Geometry: final body of the model. Coordinates: model frame, mm. Face numbers are marked on the shaded views. A direction names the side the tool comes from. Round coordinates to 2 decimals unless told otherwise and drop trailing zeros. Loops run counter-clockwise (first coordinate to the right, second up) from the corner with the lowest first, then second, coordinate; pieces in that order, holes last. Notation, with made-up numbers: (67, -22.75) -> (90, -22.75) arc R26 ccw to (90, 13.25) -> close; hole circle Ø11 at (-25.75, 60). An arc over 180 degrees is marked (long way). Answer in a Markdown table with one row per item.
```python
from build123d import *

# Parameters (mm, degrees)
SKETCH1_R           = 2.5
BOSS_EXTRUDE1_DEPTH = 15
SKETCH2_R           = 5
BOSS_EXTRUDE2_DEPTH = 3
CUT_EXTRUDE1_START  = -1.5
CUT_EXTRUDE1_DEPTH  = 1.5


with BuildPart() as part:
    # Sketch1 → Boss-Extrude1 (new body)
    with BuildSketch(Plane(origin=(0, 0, 0), x_dir=(1, 0, 0), z_dir=(0, 1, 0))):
        with Locations(Location((0, 0, 0), (0, 0, 270))):
            Circle(SKETCH1_R)
    extrude(amount=BOSS_EXTRUDE1_DEPTH)

    # Sketch2 → Boss-Extrude2 (add)
    with BuildSketch(Plane(origin=(0, 15, 0), x_dir=(1, 0, 0), z_dir=(0, 1, 0))):
        with Locations(Location((0, 0, 0), (0, 0, 270))):
            Circle(SKETCH2_R)
    extrude(amount=BOSS_EXTRUDE2_DEPTH)

    # Sketch3 → Cut-Extrude1 (cut)
    with BuildSketch(Plane(origin=(0, 18, 0), x_dir=(1, 0, 0), z_dir=(0, 1, 0)).offset(CUT_EXTRUDE1_START)):
        with BuildLine():
            Line((-1.5, 4.769696007), (-1.5, -4.769696007))
            ThreePointArc((-1.5, -4.769696007), (0, -5), (1.5, -4.769696007))
            Line((1.5, -4.769696007), (1.5, 4.769696007))
            ThreePointArc((1.5, 4.769696007), (0, 5), (-1.5, 4.769696007))
        make_face()
    extrude(amount=CUT_EXTRUDE1_DEPTH, mode=Mode.SUBTRACT)


solid = part.part
```
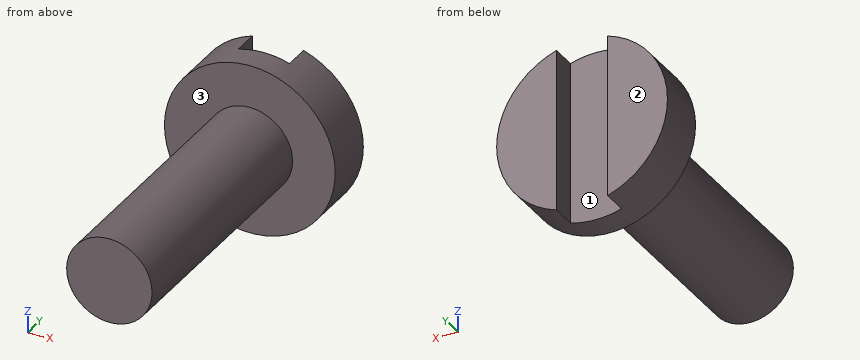
Item 1: Cut plane D-D (y = 9.5). Output: boundary loops of the cut face in (x, z).
Answer:
| item | result |
|---|---|
| outline | circle Ø5 at (0, 0) |
Item 2: Cut plane B-B (z = 3). Output: boundary loops of the cut face in (x, y).
Answer:
| item | result |
|---|---|
| outline | (-4, 15) -> (4, 15) -> (4, 18) -> (1.5, 18) -> (1.5, 16.5) -> (-1.5, 16.5) -> (-1.5, 18) -> (-4, 18) -> close |
Item 3: Cut plane C-C (y = 17.25). Output: boundary loops of the cut face in (x, z).
Answer:
| item | result |
|---|---|
| outline | (-1.5, -4.77) -> (-1.5, 4.77) arc R5 ccw to start; (1.5, -4.77) arc R5 ccw to (1.5, 4.77) -> close |
Item 4: Cut plane A-A (x = 0). Output: boundary loops of the cut face in (y, z), then the cut area to 3 significant figures.
Answer:
| item | result |
|---|---|
| outline | (0, -2.5) -> (15, -2.5) -> (15, -5) -> (16.5, -5) -> (16.5, 5) -> (15, 5) -> (15, 2.5) -> (0, 2.5) -> close |
| area | 90.0 mm² |
Item 5: Pin query (flat end, axial travel): pin 1 Ø1.5 at (x, z) = (-0.5, -2) entering from +Y; pin 2 Ø2 at (y, z) = (2, 1.5) entering from -X; pin 3 Ø1.2 at (y, z) = (17.5, -1) entering from -X. Return the tip coordinate at first contact, or that it passes through.
Answer:
| item | result |
|---|---|
| pin 1 | stops at y = 16.5 |
| pin 2 | stops at x = -2.45 |
| pin 3 | stops at x = -4.98 |
Item 6: Reachability of the marked faces 1, 2 and 3 from +Z, -Z, +X, -X, +Y, -Y: full face, straight path, thin tool, end or side. Return the list, or none.
Answer:
| item | result |
|---|---|
| face 1 | +Z, -Z, +Y |
| face 2 | +Z, -Z, +X, -X, +Y |
| face 3 | -Y |
Item 7: Line query: probe 1 along Y at (x, z) = (-3.25, -1.75); probe 2 along Y at (x, z) = (-1, -0.5); probe 3 along X at (y, z) = (14.5, 0). Output: solid intervals per line, ascending. Write a range as [from, to].
Answer:
| item | result |
|---|---|
| probe 1 | y = [15, 18] |
| probe 2 | y = [0, 16.5] |
| probe 3 | x = [-2.5, 2.5] |
